```python
from build123d import *

# Parameters (mm, degrees)
SKETCH1_R           = 1.4
BOSS_EXTRUDE1_DEPTH = 0.8


with BuildPart() as part:
    # Sketch1 → Boss-Extrude1 (new, symmetric)
    with BuildSketch(Plane(origin=(0, 0, 0), x_dir=(0, 0, -1), z_dir=(1, 0, 0))):
        with BuildLine():
            Line((-35.115, -40.115), (35.115, -40.115))
            ThreePointArc((35.115, -40.115), (38.650533906, -38.650533906), (40.115, -35.115))
            Line((40.115, -35.115), (40.115, 35.115))
            ThreePointArc((40.115, 35.115), (38.650533906, 38.650533906), (35.115, 40.115))
            Line((35.115, 40.115), (-35.115, 40.115))
            ThreePointArc((-35.115, 40.115), (-38.650533906, 38.650533906), (-40.115, 35.115))
            Line((-40.115, 35.115), (-40.115, -35.115))
            ThreePointArc((-40.115, -35.115), (-38.650533906, -38.650533906), (-35.115, -40.115))
        make_face()
        with Locations((-36.615, 26.615)):
            Circle(SKETCH1_R, mode=Mode.SUBTRACT)
        with Locations((21.384224133, 26.315)):
            Circle(SKETCH1_R, mode=Mode.SUBTRACT)
        with Locations((35.384224133, -35.385)):
            Circle(SKETCH1_R, mode=Mode.SUBTRACT)
        with Locations((-35.115, -35.385)):
            Circle(SKETCH1_R, mode=Mode.SUBTRACT)
    extrude(amount=BOSS_EXTRUDE1_DEPTH, both=True)


solid = part.part
```
Work out the finished part from the listing and answer in its coordinate system (mm). Give positions to 0.01 mm unless a question says otherwise; leave off trailing zeros. Answer as CSV lines item,"result". Start each with the question number.
(1) For a pull along Z with two mould halves and no side action, classify faces 1 (the cylindrical face through (0, -38.6, 38.7)), 2 (the cylindrical face through (-0.01, -35.92, 33.82)), 3 (the flat face through (-0.8, 1, 1)), 4 (the cylindrical face through (0, -38.7, -38.6)) as released by +Z, released by -Z, zero draft, split by the parting line, or undercut.
(2) This flat-tipped pin is pushed along its axis until it touches: pin 1 Ø3.5 at (y, z) = (26.615, 36.615) entering from -X. Where does it stop, or does it pass through?
(3) Consider line 1 along Z through (x, y) = (0.4, 26.5) (1 decimal); line 2 along Y through (x, z) = (-0.6, -21.5) (3 decimals); line 3 along Z through (x, y) = (0.7, -34.5) (3 decimals). Determine where each line is inside the solid, lowest interval first.
Entries:
1,face 1,"released by +Z"
1,face 2,"undercut"
1,face 3,"zero draft"
1,face 4,"released by -Z"
2,pin 1,"x = -0.8"
3,line 1,"-40.1 to -22.8, -20 to 35.2, 38 to 40.1"
3,line 2,"-40.115 to 24.92, 27.71 to 40.115"
3,line 3,"-40.115 to -36.469, -34.299 to 34.03, 36.2 to 40.115"
